Input: part model. Units: mm. Frame: model coordinates. Face numbers are marked on the shaded views. A direction names the side the tool comes from. Coordinates: 2 decimals unless noted, no trailing zeros. Loops run counter-clockwise (first coordinate to the right, second up) from the corner with the lowest first, then second, coordinate; pieces in that order, holes last. Notation, with made-up numbers: (85, -17) - (135, -17) arc R26 ccw to (135, 10) - close; hole circle Ø8 at (81, 37.25). An arc over 180 degrees is marked (long way). Use one line per item in the form item = value.
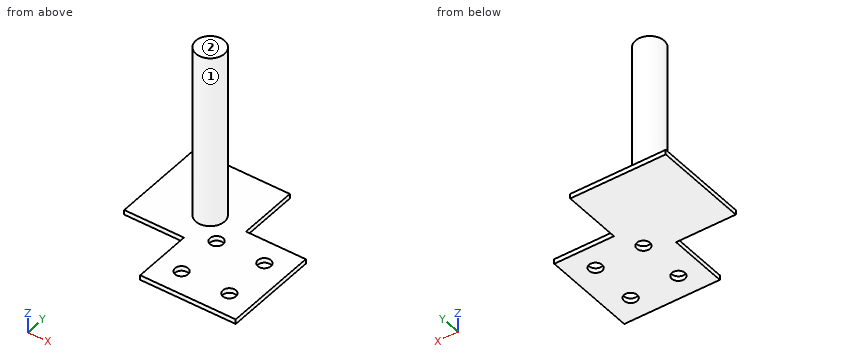
from build123d import *

# Parameters (mm, degrees)
F0_R     = 5.5
F0_R_2   = 12
F1_DEPTH = 4
F2_R     = 12
F3_DEPTH = 150


with BuildPart() as f1:
    # F0 (on Top) → F1 (new body)
    with BuildSketch(Plane.XY):
        Polygon((30, 50), (-50, 50), (-50, -30), (0, -30), (0, -80), (80, -80), (80, 0), (30, 0), align=None)
        with Locations((20, -60)):
            Circle(F0_R, mode=Mode.SUBTRACT)
        with Locations((60, -60)):
            Circle(F0_R, mode=Mode.SUBTRACT)
        with Locations((20, -20)):
            Circle(F0_R, mode=Mode.SUBTRACT)
        with Locations((60, -20)):
            Circle(F0_R, mode=Mode.SUBTRACT)
        Circle(F0_R_2, mode=Mode.SUBTRACT)
    extrude(amount=F1_DEPTH)

    # F2 (on face) → F3 (join)
    with BuildSketch(Plane(origin=(0, 0, 0), x_dir=(1, 0, 0), z_dir=(0, 0, -1))):
        Circle(F2_R)
    extrude(amount=-F3_DEPTH)


solid = f1.part
Q1. Ray query, line 1 along Y through (x, z) = (60, 2.8); line 2 along Y through (x, z) = (20, 1.2); line 3 along Z through (x, y) = (58.5, -40.5). Return the intervals inside material, ascending. Write a range as [from, to].
Check values:
line_1 = [-80, -65.5], [-54.5, -25.5], [-14.5, 0]
line_2 = [-80, -65.5], [-54.5, -25.5], [-14.5, 50]
line_3 = [0, 4]
Q2. Set-up query: the marked faces 1 and 2. Return all of +Z, -Z, +X, -X, +Y, -Y with unobstructed straight access to the full face (end or side cutting, diameter ignored); none if empty.
Check values:
face_1 = +Z
face_2 = +Z, +X, -X, +Y, -Y
Q3. Cut plane A-A, the plane y = -20. Return loops of the section in (x, z).
Check values:
outline = (-50, 0) - (14.5, 0) - (14.5, 4) - (-50, 4) - close; (25.5, 0) - (54.5, 0) - (54.5, 4) - (25.5, 4) - close; (65.5, 0) - (80, 0) - (80, 4) - (65.5, 4) - close
Q4. Cut plane D-D, the plane x = -39. Return loops of the section in (y, z), then the cut area to 3 significant figures.
Check values:
outline = (-30, 0) - (50, 0) - (50, 4) - (-30, 4) - close
area = 320 mm²
Q5. Cut plane C-C, the plane z = 13. Return loops of the section in (x, y).
Check values:
outline = circle Ø24 at (0, 0)
Q6. First-contact query: P1, Ø4.5, axis at x = 66.5, z = 2.5, coming from the +Y side; P2, Ø8, axis at x = 1, y = 26.5, coming from the +Z side; P3, Ø9, axis at x = 20, y = -20, coming from the +Z side; P4, Ø3, axis at x = -14.5, z = 3, coming from the -Y side. Flat tips, straight axial feed; report the tip coordinate or a pass-through.
Check values:
P1 = 0
P2 = 4
P3 = through
P4 = -30
Q7. Cut plane B-B, the plane x = 60. Return loops of the section in (y, z), then the cut area to 3 significant figures.
Check values:
outline = (-80, 0) - (-65.5, 0) - (-65.5, 4) - (-80, 4) - close; (-54.5, 0) - (-25.5, 0) - (-25.5, 4) - (-54.5, 4) - close; (-14.5, 0) - (0, 0) - (0, 4) - (-14.5, 4) - close
area = 232 mm²
